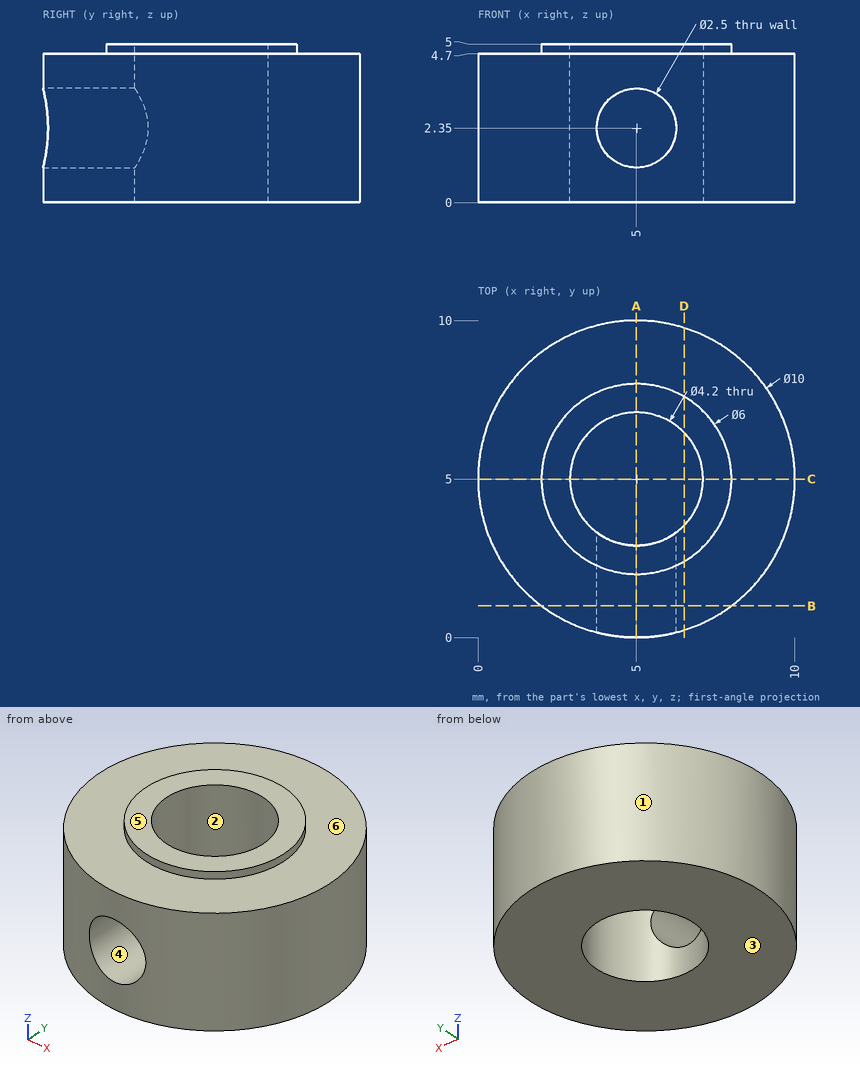
Verification items for this drawing (mm, ordinates from the low corner). A direction names the side the tool comes from. Coordinates: 2 decimals unless noted, no trailing zeros. Order: outer loops, then holes, each group sorted by start corner. A loop starts at its lowest first (then second) coordinate and runs counter-clockwise, first axis right, second up. Notation, with made-up numbers: (47.25, 41.25) -> (68.25, 41.25) arc R10 ccw to (68.25, 54.25) -> close; hole circle Ø6 at (-21.75, -26.75). An arc over 180 degrees is marked (long way). Put each result on its own line as item: value. Start each with the question number.
1. Material ranges on L1, parallel to Z at x = 1, y = 4.5; L2, parallel to X at y = 6, z = 2.15; L3, parallel to X at y = 4.75, z = 0.35, recorded low to high. Write a range as [from, to].
2. Cross-section at C-C, the plane y = 5. Record the boundary of the cut face in (x, z), then the cut area to 3 significant figures.
3. Access from +Z, -Z, +X, -X, +Y, -Y to the whole of each face (thin tool, end or side, straight path). Record for the marked faces 4, 5 and 6.
4. Cross-section at D-D, the plane x = 6.5. Record the boundary of the cut face in (y, z), then the cut area to 3 significant figures.
5. Go/stop test with flat-tipped pins: pin 1 Ø2 at (x, z) = (5, 2.35) entering from -Y; pin 2 Ø3 at (y, z) = (8, 4) entering from +X; pin 3 Ø2.5 at (x, y) = (5, 5) entering from +Z; pin 4 Ø1.5 at (x, z) = (4, 1.5) entering from -Y. Record where each tip stops, or that it passes through.
6. Mould release check, pull along X, two halves, no side actions. Record for the marked faces 1, 2 and 3: released by +X, released by -X, zero draft, split by the parting line, or undercut.
7. Cross-section at B-B, the plane y = 1. Record the boundary of the cut face in (x, z).
8. Cross-section at A-A, the plane x = 5. Record the boundary of the cut face in (y, z).
Computed:
1. L1: [0, 4.7]
1. L2: [0.1, 3.15], [6.85, 9.9]
1. L3: [0.01, 2.91], [7.09, 9.99]
2. outline: (0, 0) -> (2.9, 0) -> (2.9, 5) -> (2, 5) -> (2, 4.7) -> (0, 4.7) -> close; (7.1, 0) -> (10, 0) -> (10, 4.7) -> (8, 4.7) -> (8, 5) -> (7.1, 5) -> close
2. area: 27.8 mm2
3. face 4: -Y
3. face 5: +Z, +X, -X, +Y, -Y
3. face 6: +Z
4. outline: (0.23, 0) -> (3.53, 0) -> (3.53, 5) -> (2.4, 5) -> (2.4, 4.7) -> (0.23, 4.7) -> close; (6.47, 0) -> (9.77, 0) -> (9.77, 4.7) -> (7.6, 4.7) -> (7.6, 5) -> (6.47, 5) -> close
4. area: 31.7 mm2
5. pin 1: y = 6.85
5. pin 2: x = 9.77
5. pin 3: through
5. pin 4: y = 0.01
6. face 1: split by the parting line
6. face 2: undercut
6. face 3: zero draft
7. outline: (2, 0) -> (8, 0) -> (8, 4.7) -> (2, 4.7) -> close; hole circle Ø2.5 at (5, 2.35)
8. outline: (0, 0) -> (2.9, 0) -> (2.9, 1.1) -> (0, 1.1) -> close; (0, 3.6) -> (2.9, 3.6) -> (2.9, 5) -> (2, 5) -> (2, 4.7) -> (0, 4.7) -> close; (7.1, 0) -> (10, 0) -> (10, 4.7) -> (8, 4.7) -> (8, 5) -> (7.1, 5) -> close
